from build123d import *

# Parameters (mm, degrees)
BASPROSKE_W             = 5
BASPROSKE_H             = 6.5
TOOTHCUT_DEPTH          = 11.464224768
TEETHCUTS_COUNT         = 11
TEETHCUTS_ANGLE         = 327.272727273
BORSKE_R                = 1.5
BORE_DEPTH              = 50.0000508
ESQUISSE1_R             = 2.75
ENL_V_MAT_EXTRU_1_DEPTH = 3


with BuildPart() as part:
    # BasProSke → Base-Revolve (revolve)
    with BuildSketch(Plane(origin=(0, 0, 0), x_dir=(1, 0, 0), z_dir=(0, 1, 0)), mode=Mode.PRIVATE) as base_revolve_sk:
        with Locations((2.5, 3.25)):
            Rectangle(BASPROSKE_W, BASPROSKE_H)
    revolve(base_revolve_sk.sketch.rotate(Axis((-10, 0, 0), (1, 0, 0)), 180), axis=Axis((-10, 0, 0), (1, 0, 0)))

    # TooCutSke → ToothCut (cut, through all)
    with BuildSketch(Plane(origin=(0, 0, 0), x_dir=(0, 0, -1), z_dir=(1, 0, 0))):
        with BuildLine():
            ThreePointArc((0.576045815, 4.209771041), (0, 4.249), (-0.576045815, 4.209771041))
            ThreePointArc((-0.576045815, 4.209771041), (-0.841371334, 5.420048739), (-1.718652745, 6.295004202))
            ThreePointArc((-1.718652745, 6.295004202), (0, 6.5254), (1.718652745, 6.295004202))
            ThreePointArc((1.718652745, 6.295004202), (0.841371334, 5.420048739), (0.576045815, 4.209771041))
        make_face()
    toothcut = extrude(amount=TOOTHCUT_DEPTH, mode=Mode.SUBTRACT)

    # TeethCuts: ToothCut ×11 about axis
    teethcuts_axis = Axis((-10, 0, 0), (1, 0, 0))
    for i in range(1, TEETHCUTS_COUNT):
        add(toothcut.rotate(teethcuts_axis, i * TEETHCUTS_ANGLE / (TEETHCUTS_COUNT - 1)), mode=Mode.SUBTRACT)

    # BorSke → Bore (cut, symmetric)
    with BuildSketch(Plane(origin=(0, 0, 0), x_dir=(0, 0, -1), z_dir=(1, 0, 0))):
        with Locations(Location((0, 0, 0), (0, 0, 180))):
            Circle(BORSKE_R)
    extrude(amount=BORE_DEPTH, both=True, mode=Mode.SUBTRACT)

    # Esquisse1 → Enlèv. mat.-Extru.1 (cut)
    with BuildSketch(Plane.ZY):
        Circle(ESQUISSE1_R)
    extrude(amount=-ENL_V_MAT_EXTRU_1_DEPTH, mode=Mode.SUBTRACT)


solid = part.part
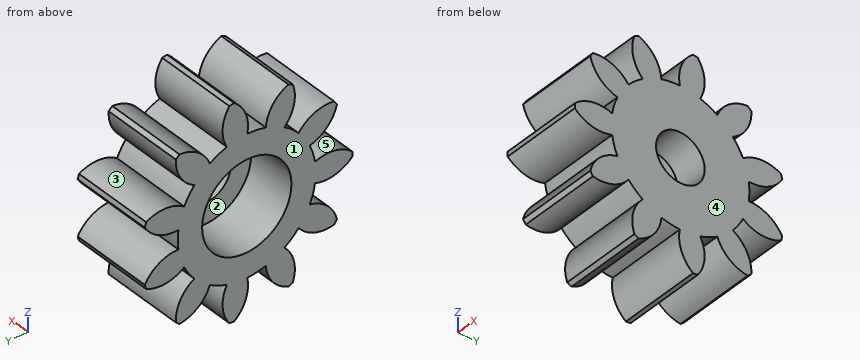
For this review, take the finished solid that the model builds, in its own axes (mm). Face numbers are marked on the shaded views. A direction names the side the tool comes from. Give positions to 0.01 mm unless a question says otherwise; leave off trailing zeros. Order: outer loops, then holes, each group sorted by start corner. A loop starts at its lowest first (then second) coordinate and runs counter-clockwise, first axis right, second up. Notation, with made-up numbers: M 18.25,-37.75 L 39.25,-37.75 A13 ccw 39.25,-24.75 Z; hole C 33,5 d8. An arc over 180 degrees is marked long. Answer in a Markdown table with one row per item. Add a question column.
(1) Consider section D-D on z = -2.5. State the section outline as (x, y) points, and give its area (3 significant figures).
(2) For the marked faces 1, 2 and 3, list the 3-axis set-ups (+Z, -Z, +X, -X, +Y, -Y) from which the entire face can be reached by the end or side of a thin tool; tool diameter is ignored.
(3) Wall thickness on probe 1 along Y at (x, z) = (4.25, -3.5); probe 2 along Z at (x, y) = (0.35, 0.75); probe 3 along Y at (x, z) = (3.6, 1): over which ranges is each line inside the solid? List them lowest first. Write a range as [from, to].
(4) For pin 1 (3 mm diameter, centred on x = 1.5, y = 2.5, fed in from -Z); pin 2 (2.5 mm diameter, centred on y = 0, z = 0, fed in from -X); pin 3 (1.5 mm diameter, centred on x = 3, y = 2, fed in from -Z); pin 4 (3.5 mm diameter, centred on y = 0, z = 0, fed in from -X), all flat-tipped, find the tip position at first contact; note any pin that passes through.
(5) Consider section B-B on y = -4.75. State the section outline as (x, z) points.
(6) Consider section C-C on y = -0.75. State the section outline as (x, z) points, and give its area (3 significant figures).
(7) Mouldability with a two-part tool opening along Y and no side actions: class the marked faces 4 and 5 as +Y half, -Y half, draft (parallel to the pull), parting line (faces both ways), or undercut.
(8) Consider section A-A on z = 3. State the section outline as (x, y) points.
Evaluation:
| question | item | result |
|---|---|---|
| 1 | outline | M 0,-5.11 L 5,-5.11 L 5,3.44 L 0,3.44 L 0,1.15 L 3,1.15 L 3,-1.15 L 0,-1.15 Z |
| 1 | area | 35.9 mm^2 |
| 2 | face 1 | +Z, -Z, -X, +Y, -Y |
| 2 | face 2 | -X |
| 2 | face 3 | +X, -X |
| 3 | probe 1 | y = [-5.48, -4.07], [-2.41, 4.02] |
| 3 | probe 2 | z = [-6.43, -2.65], [2.65, 6.43] |
| 3 | probe 3 | y = [-4.13, -1.12], [1.12, 5.67] |
| 4 | pin 1 | stops at z = -6.42 |
| 4 | pin 2 | passes through |
| 4 | pin 3 | stops at z = -6.12 |
| 4 | pin 4 | stops at x = 3 |
| 5 | outline | M 0,-3.67 L 5,-3.67 L 5,-2.15 L 0,-2.15 Z; M 0,-0.76 L 5,-0.76 L 5,0.76 L 0,0.76 Z; M 0,2.15 L 5,2.15 L 5,3.67 L 0,3.67 Z |
| 6 | outline | M 0,-4.18 L 5,-4.18 L 5,-1.3 L 3,-1.3 L 3,-2.65 L 0,-2.65 Z; M 0,2.65 L 3,2.65 L 3,1.3 L 5,1.3 L 5,4.18 L 0,4.18 Z |
| 6 | area | 20.8 mm^2 |
| 7 | face 4 | draft |
| 7 | face 5 | undercut |
| 8 | outline | M 0,-5.42 L 5,-5.42 L 5,-3.36 L 0,-3.36 Z; M 0,-3.01 L 5,-3.01 L 5,3.58 L 0,3.58 Z |
